Build history of the part. All positions in model axes, mm. A direction names the side the tool comes from. Coordinates: 2 decimals unless noted, no trailing zeros.
```python
from build123d import *

# Parameters (mm, degrees)
BOSS_EXTRUDE1_DEPTH = 15
CUT_EXTRUDE1_REACH  = 87.865
SKETCH3_R           = 2.1
CUT_EXTRUDE2_DEPTH  = 8
SKETCH5_R           = 2.05
CUT_EXTRUDE3_DEPTH  = 16
SKETCH5_3_R         = 4
SKETCH5_3_R_2       = 2.05
CUT_EXTRUDE4_DEPTH  = 3
SKETCH6_R           = 2.05
CUT_EXTRUDE5_DEPTH  = 2.2
FILLET1_R           = 2
SKETCH7_W           = 4
SKETCH7_H           = 4.1
CUT_EXTRUDE6_DEPTH  = 4.2
FILLET2_R           = 0.5


with BuildPart() as part:
    # Sketch2 → Boss-Extrude1 (new body)
    with BuildSketch(Plane(origin=(0, 0, 0), x_dir=(0, 0, -1), z_dir=(1, 0, 0))):
        with BuildLine():
            ThreePointArc((182.713463258, 0), (188.370317508, 2.343145751), (190.713463258, 8))
            Line((190.713463258, 8), (190.713463258, 60.22857568))
            Line((190.713463258, 60.22857568), (182.203249602, 87.327423803))
            Line((182.203249602, 87.327423803), (10.472480761, 33.39651399))
            Line((10.472480761, 33.39651399), (19.096918934, 5.933943762))
            Line((19.096918934, 5.933943762), (24.551301688, 0))
            Line((24.551301688, 0), (182.713463258, 0))
        make_face()
        with BuildLine():
            Line((37.938354626, 26.299705178), (165.973133125, 66.508178818))
            ThreePointArc((165.973133125, 66.508178818), (170.547399424, 66.102716631), (173.49518908, 62.58151685))
            Line((173.49518908, 62.58151685), (175.43782222, 56.395641556))
            ThreePointArc((175.43782222, 56.395641556), (175.644152669, 55.507297693), (175.713463258, 54.597944563))
            Line((175.713463258, 54.597944563), (175.713463258, 21.281778339))
            ThreePointArc((175.713463258, 21.281778339), (173.956103945, 17.039137651), (169.713463258, 15.281778339))
            Line((169.713463258, 15.281778339), (38.483983749, 15.281778339))
            ThreePointArc((38.483983749, 15.281778339), (33.847693688, 20.428280139), (37.659397671, 26.212100595))
            ThreePointArc((37.659397671, 26.212100595), (37.798310715, 26.257703381), (37.938354626, 26.299705178))
        make_face(mode=Mode.SUBTRACT)
    extrude(amount=BOSS_EXTRUDE1_DEPTH)

    # Sketch3 → Cut-Extrude1 (cut, up to next)
    with BuildSketch(Plane(origin=(0, 27.404937127, 8.606338879), x_dir=(1, 0, 0), z_dir=(0, 0.954059827, 0.299616166)), mode=Mode.PRIVATE) as cut_extrude1_sk1:
        with Locations((7.5, 170.997508649)):
            Circle(SKETCH3_R)
    cut_extrude1_tool1 = extrude(cut_extrude1_sk1.sketch, amount=-CUT_EXTRUDE1_REACH, mode=Mode.PRIVATE) & part.part
    add(cut_extrude1_tool1.solids().sort_by_distance((7.5, 78.638555, -154.535515))[0], mode=Mode.SUBTRACT)
    # Sketch3 → Cut-Extrude1 (cut, up to next)
    with BuildSketch(Plane(origin=(0, 27.404937127, 8.606338879), x_dir=(1, 0, 0), z_dir=(0, 0.954059827, 0.299616166)), mode=Mode.PRIVATE) as cut_extrude1_sk2:
        with Locations((7.5, 50.997508649)):
            Circle(SKETCH3_R)
    cut_extrude1_tool2 = extrude(cut_extrude1_sk2.sketch, amount=-CUT_EXTRUDE1_REACH, mode=Mode.PRIVATE) & part.part
    add(cut_extrude1_tool2.solids().sort_by_distance((7.5, 42.684615, -40.048335))[0], mode=Mode.SUBTRACT)

    # Sketch4 → Cut-Extrude2 (cut)
    with BuildSketch(Plane(origin=(0, 13.094039723, 4.112096395), x_dir=(1, 0, 0), z_dir=(0, -0.954059827, -0.299616166))):
        Polygon((3.910348885, -172.976836364), (7.419322526, -175.095901563), (11.008973641, -173.116573848), (11.089651115, -169.018180934), (7.580677474, -166.899115735), (3.991026359, -168.87844345), align=None)
        Polygon((7.302343544, -46.903089855), (3.855301083, -49.121474764), (4.052957539, -53.215893558), (7.697656456, -55.091927443), (11.144698917, -52.873542534), (10.947042461, -48.77912374), align=None)
    extrude(amount=-CUT_EXTRUDE2_DEPTH, mode=Mode.SUBTRACT)

    # Sketch5 → Cut-Extrude3 (cut, through all)
    with BuildSketch(Plane.ZY):
        with Locations((-178.166164975, 73.481776555)):
            Circle(SKETCH5_R)
        with Locations((-182.713463258, 8)):
            Circle(SKETCH5_R)
        with Locations((-21.700353364, 24.344725393)):
            Circle(SKETCH5_R)
    extrude(amount=-CUT_EXTRUDE3_DEPTH, mode=Mode.SUBTRACT)

    # Sketch5_3 → Cut-Extrude4 (cut)
    with BuildSketch(Plane.ZY):
        with Locations((-178.166164975, 73.481776555)):
            Circle(SKETCH5_3_R)
        with Locations((-182.713463258, 8)):
            Circle(SKETCH5_3_R)
        with Locations((-182.713463258, 8)):
            Circle(SKETCH5_3_R_2, mode=Mode.SUBTRACT)
        with Locations((-21.700353364, 24.344725393)):
            Circle(SKETCH5_3_R)
    extrude(amount=-CUT_EXTRUDE4_DEPTH, mode=Mode.SUBTRACT)

    # Sketch6 → Cut-Extrude5 (cut)
    with BuildSketch(Plane(origin=(15, 0, 0), x_dir=(0, 0, -1), z_dir=(1, 0, 0))):
        with Locations((24.69651502, 14.804127124)):
            Circle(SKETCH6_R)
        with Locations((181.162326631, 63.941178286)):
            Circle(SKETCH6_R)
    extrude(amount=-CUT_EXTRUDE5_DEPTH, mode=Mode.SUBTRACT)

    # Fillet1
    fillet1_edges = [part.edges().sort_by_distance(p)[0] for p in [
        (15, 46.403941998, -101.955743876),
        (15, 66.102716631, -170.547399424),
        (0, 2.966971881, -21.824110311),
        (0, 19.665228876, -14.784699847),
        (0, 73.777999741, -186.45835643),
        (0, 34.11428784, -190.713463258),
        (0, 2.343145751, -188.370317508),
        (0, 0, -103.632382473),
        (0, 15.281778339, -104.098723504),
        (0, 17.039137651, -173.956103945),
        (0, 37.939861451, -175.713463258),
        (15, 59.488579203, -174.46650565),
        (0, 55.507297693, -175.644152669),
        (0, 59.488579203, -174.46650565),
        (0, 66.102716631, -170.547399424),
        (0, 46.403941998, -101.955743876),
        (0, 20.574202547, -33.838577822),
        (15, 55.507297693, -175.644152669),
        (7.5, 15.281778339, -38.483983749),
        (15, 37.939861451, -175.713463258),
        (15, 17.039137651, -173.956103945),
        (15, 15.281778339, -104.098723504),
        (15, 0, -103.632382473),
        (15, 2.343145751, -188.370317508),
        (15, 34.11428784, -190.713463258),
        (15, 20.574202547, -33.838577822),
        (15, 2.966971881, -21.824110311),
    ]]
    fillet(fillet1_edges, radius=FILLET1_R)

    # Sketch7 → Cut-Extrude6 (cut)
    with BuildSketch(Plane(origin=(15, 0, 0), x_dir=(0, 0, -1), z_dir=(1, 0, 0))):
        with Locations((182.713463258, 35.95)):
            Rectangle(SKETCH7_W, SKETCH7_H)
    extrude(amount=-CUT_EXTRUDE6_DEPTH, mode=Mode.SUBTRACT)

    # Fillet2
    fillet2_edges = [part.edges().sort_by_distance(p)[0] for p in [
        (15, 33.9, -182.713463258),
        (10.8, 35.95, -180.713463258),
        (15, 35.95, -184.713463258),
        (10.8, 33.9, -182.713463258),
        (10.8, 38, -182.713463258),
        (10.8, 35.95, -184.713463258),
        (15, 35.95, -180.713463258),
    ]]
    fillet(fillet2_edges, radius=FILLET2_R)


solid = part.part
```
1. Mould opens along Y. For faces 1 (the face through (7.423, 2.281, -188.308)), 2 (the face through (0.57, 73.787, -185.825)), 3 (the face through (7.423, 59.532, -174.453)) say: +Y half, -Y half, draft (parallel to the pull), parting line (faces both ways), or undercut.
Computed values:
face 1: -Y half
face 2: +Y half
face 3: undercut
2. Saw through at A-A on y = 31.5. State how many separate pieces and enclosed holes the cut face has, plus the area to 3 significant figures.
Computed values:
separate pieces: 2
enclosed holes: 1
area: 821 mm2
3. 3-axis set-ups, long thin cutter, end or side, ignore diameter. For faces 4 (the face through (9.189, 69.026, -160.827)), 5 (the face through (7, 15.282, -105)), 6 (the face through (1.5, 76.2, -181.1)), 7 (the face through (13.92, 16.53, -25.8)): which of +Z, -Z, +X, -X, +Y, -Y reach the whole face in a straight line?
Computed values:
face 4: none
face 5: +X, -X
face 6: -X
face 7: +X
4. Flat gauge pins, fed straight in: pin 1 (1 mm diameter, centred on x = 9, z = -92, fed in from +Y); pin 2 (2 mm diameter, centred on y = 15.5, z = -25, fed in from +X); pin 3 (5.5 mm diameter, centred on x = 5, z = -114, fed in from +Y). Where does each tip first touch, or does it go through?
Computed values:
pin 1: stops at y = 59.16
pin 2: stops at x = 12.8
pin 3: stops at y = 66.77
5. Probe line 1 along Z through (x, y) = (1.25, 25); line 2 along Z through (x, y) = (10.75, 26); line 3 along Y through (x, z) = (9.25, -119). List the from-to ranges inside material, lowest first.
Computed values:
line 1: z = -190.57 to -175.86, -35.43 to -25.65, -17.75 to -13.26
line 2: z = -190.71 to -175.71, -37.13 to -22.91, -20.49 to -12.8
line 3: y = 0 to 15.28, 51.76 to 67.48
